Design review of the part built by this model. Coordinates are the model's own, in mm. Give positions to 0.01 mm unless a question says otherwise; leave off trailing zeros. Loops run counter-clockwise (first coordinate to the right, second up) from the corner with the lowest first, then second, coordinate; pieces in that order, holes last. Notation, with made-up numbers: (-15, 36) -> (-10, 36) arc R18 ccw to (-10, 49) -> close; hole circle Ø4 at (-26.5, 3.5). An arc over 180 degrees is marked (long way). Answer in a Markdown table with one row per item. Add a question column.
(1) Consider section B-B on y = 43. Write out the cut boundary in (x, z), then the cut area to 3 significant figures.
(2) Consider section A-A on z = 39.5. Write out the cut boundary in (x, y).
(3) For line 1 (X direction, y = 23, z = 45); line 2 (X direction, y = 28, z = 38); line 3 (X direction, y = 32, z = 39), list the stretches that pass through material, from the lowest coordinate up.
(4) Consider section D-D on y = 27. Write out the cut boundary in (x, z).
(5) Draft analysis for pull direction Y (two halves, no side actions). For faces 1 (the cylindrical face through (-37.19, 24.92, 28.57)), 2 (the cylindrical face through (-10.06, 20.86, 31.1)), 3 (the flat face through (-37, 0, 27)), state which applies: +Y half, -Y half, draft (parallel to the pull), parting line (faces both ways), or undercut.
(6) For pin 1 (6 mm diameter, centred on x = -64.42, y = 25.27, fed in from +Z); pin 2 (4 mm diameter, centred on x = -41, y = 18, fed in from +Z); pin 3 (3 mm diameter, centred on x = -24.5, y = 26, fed in from +Z), all flat-tipped, find the tip position at first contact; note any pin that passes through.
(7) Consider section C-C on z = 46. Write out the cut boundary in (x, y), then the cut area to 3 significant figures.
from build123d import *

# Parameters (mm, degrees)
F0_W     = 66.982273
F0_H     = 39.254546
F1_DEPTH = 50.546
F3_DEPTH = 60.198
F4_R     = 3.641507
F4_R_2   = 3.822226
F5_DEPTH = 136.652


with BuildPart() as f1:
    # F0 (on Front) → F1 (new body)
    with BuildSketch(Plane.XZ):
        with Locations((-36.711974, 30.826364)):
            Rectangle(F0_W, F0_H)
    extrude(amount=-F1_DEPTH)

    # F2 (on face) → F3 (cut)
    with BuildSketch(Plane.XZ):
        with BuildLine():
            ThreePointArc((-58.599127, 50.453637), (-36.711974, 28.566484), (-14.824822, 50.453637))
            Line((-14.824822, 50.453637), (-58.599127, 50.453637))
        make_face()
        with BuildLine():
            Line((-58.599127, 50.453637), (-14.824822, 50.453637))
            ThreePointArc((-14.824822, 50.453637), (-36.711974, 72.34079), (-58.599127, 50.453637))
        make_face()
    extrude(amount=-F3_DEPTH, mode=Mode.SUBTRACT)

    # F4 (on face) → F5 (cut)
    with BuildSketch(Plane.XY.offset(50.453637)):
        with Locations((-64.423636, 25.273)):
            Circle(F4_R)
        with Locations((-9.236364, 24.591818)):
            Circle(F4_R_2)
    extrude(amount=-F5_DEPTH, mode=Mode.SUBTRACT)


solid = f1.part
Values follow:
| question | item | result |
|---|---|---|
| 1 | outline | (-70.2, 11.2) -> (-3.22, 11.2) -> (-3.22, 50.45) -> (-14.82, 50.45) arc R21.89 cw to (-58.6, 50.45) -> (-70.2, 50.45) -> close |
| 1 | area | 1,880 mm2 |
| 2 | outline | (-70.2, 0) -> (-55.66, 0) -> (-55.66, 50.55) -> (-70.2, 50.55) -> close; (-17.76, 0) -> (-3.22, 0) -> (-3.22, 50.55) -> (-17.76, 50.55) -> close; hole circle Ø7.28 at (-64.42, 25.27); hole circle Ø7.64 at (-9.24, 24.59) |
| 3 | line 1 | -70.2 to -67.27, -61.58 to -57.91, -15.52 to -12.71, -5.76 to -3.22 |
| 3 | line 2 | -70.2 to -66.84, -62.01 to -54.71, -18.71 to -10.97, -7.51 to -3.22 |
| 3 | line 3 | -70.2 to -55.36, -18.06 to -3.22 |
| 4 | outline | (-70.2, 11.2) -> (-67.63, 11.2) -> (-67.63, 50.45) -> (-70.2, 50.45) -> close; (-61.22, 11.2) -> (-12.2, 11.2) -> (-12.2, 50.45) -> (-14.82, 50.45) arc R21.89 cw to (-58.6, 50.45) -> (-61.22, 50.45) -> close; (-6.27, 11.2) -> (-3.22, 11.2) -> (-3.22, 50.45) -> (-6.27, 50.45) -> close |
| 5 | face 1 | draft |
| 5 | face 2 | undercut |
| 5 | face 3 | -Y half |
| 6 | pin 1 | through |
| 6 | pin 2 | z = 29.49 |
| 6 | pin 3 | z = 33.39 |
| 7 | outline | (-70.2, 0) -> (-58.14, 0) -> (-58.14, 50.55) -> (-70.2, 50.55) -> close; (-15.28, 0) -> (-3.22, 0) -> (-3.22, 50.55) -> (-15.28, 50.55) -> close; hole circle Ø7.28 at (-64.42, 25.27); hole circle Ø7.64 at (-9.24, 24.59) |
| 7 | area | 1,130 mm2 |
